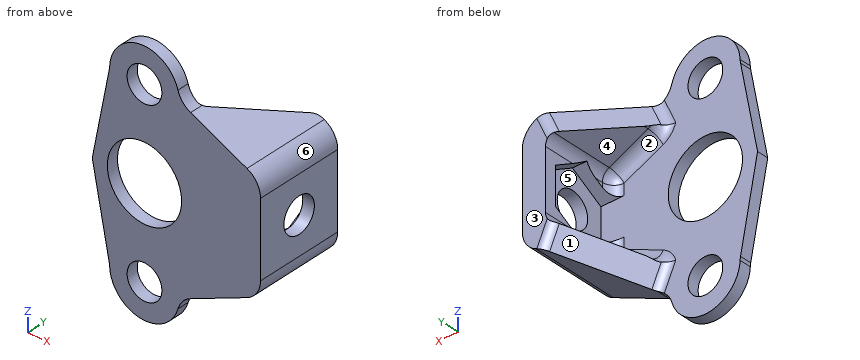
from build123d import *

# Parameters (mm, degrees)
ESQUISSE1_R                  = 3.2
ESQUISSE1_R_2                = 1.5
BOSS_EXTRU_1_DEPTH           = 1
BOSS_EXTRU_2_START           = 6.6
BOSS_EXTRU_2_DEPTH           = 6.6
CHANFREIN1_SIZE              = 6.6
CHANFREIN1_SIZE_2            = 4.73
CONG_1_R                     = 1
ENL_V_MAT_EXTRU_1_DEPTH      = 18.728508153
ENL_V_MAT_EXTRU_1_DEPTH_BACK = 1
ENL_V_MAT_EXTRU_2_DEPTH      = 18.728508153
ENL_V_MAT_EXTRU_2_DEPTH_BACK = 18.728508153
ESQUISSE2_3_R                = 1.5


with BuildPart() as part:
    # Esquisse1 → Boss.-Extru.1 (new body)
    # profile 1 of 2: a face of its own
    with BuildSketch(Plane(origin=(0, 0, 0), x_dir=(1, 0, 0), z_dir=(0, 1, 0))):
        with BuildLine():
            Line((7.41575976, 3.482294806), (4.054342249, 5.018942811))
            ThreePointArc((4.054342249, 5.018942811), (3.533019895, 5.579308264), (3.560627534, 6.344177047))
            Line((3.560627534, 6.344177047), (3.976387294, 7.253651523))
            ThreePointArc((3.976387294, 7.253651523), (3.291254041, 7.768850358), (2.884744089, 8.523560284))
            ThreePointArc((2.884744089, 8.523560284), (-0.351141019, 10.679379127), (-2.997167453, 7.830335178))
            ThreePointArc((-2.997167453, 7.830335178), (-3.009169797, 7.681917242), (-3.032181114, 7.534803614))
            Line((-3.032181114, 7.534803614), (-4.5, 0))
            Line((-4.5, 0), (-3.032181114, -7.534803614))
            ThreePointArc((-3.032181114, -7.534803614), (-3.009169797, -7.681917242), (-2.997167453, -7.830335178))
            ThreePointArc((-2.997167453, -7.830335178), (-0.351141019, -10.679379127), (2.884744089, -8.523560284))
            ThreePointArc((2.884744089, -8.523560284), (3.291254041, -7.768850358), (3.976387294, -7.253651523))
            Line((3.976387294, -7.253651523), (3.560627534, -6.344177047))
            ThreePointArc((3.560627534, -6.344177047), (3.533019895, -5.579308264), (4.054342249, -5.018942811))
            Line((4.054342249, -5.018942811), (7.41575976, -3.482294806))
            ThreePointArc((7.41575976, -3.482294806), (7.841355977, -3.113301708), (8, -2.572820331))
            Line((8, -2.572820331), (8, 2.572820331))
            ThreePointArc((8, 2.572820331), (7.841355977, 3.113301708), (7.41575976, 3.482294806))
        make_face()
        with Locations(Location((0, 0, 0), (0, 0, 270))):
            Circle(ESQUISSE1_R, mode=Mode.SUBTRACT)
        with Locations(Location((0, 7.7, 0), (0, 0, 270))):
            Circle(ESQUISSE1_R_2, mode=Mode.SUBTRACT)
        with Locations(Location((0, -7.7, 0), (0, 0, 270))):
            Circle(ESQUISSE1_R_2, mode=Mode.SUBTRACT)
    # profile 2 of 2: a face of its own
    with BuildSketch(Plane(origin=(0, 0, 0), x_dir=(1, 0, 0), z_dir=(0, 1, 0))):
        with BuildLine():
            ThreePointArc((4.054342249, 5.018942811), (3.533019895, 5.579308264), (3.560627534, 6.344177047))
            Line((3.560627534, 6.344177047), (3.976387294, 7.253651523))
            Line((3.976387294, 7.253651523), (8.831519521, 5.034162505))
            ThreePointArc((8.831519521, 5.034162505), (9.682711954, 4.29617631), (10, 3.215213554))
            Line((10, 3.215213554), (10, -3.215213554))
            ThreePointArc((10, -3.215213554), (9.682711954, -4.29617631), (8.831519521, -5.034162505))
            Line((8.831519521, -5.034162505), (3.976387294, -7.253651523))
            Line((3.976387294, -7.253651523), (3.560627534, -6.344177047))
            ThreePointArc((3.560627534, -6.344177047), (3.533019895, -5.579308264), (4.054342249, -5.018942811))
            Line((4.054342249, -5.018942811), (7.41575976, -3.482294806))
            ThreePointArc((7.41575976, -3.482294806), (7.841355977, -3.113301708), (8, -2.572820331))
            Line((8, -2.572820331), (8, 2.572820331))
            ThreePointArc((8, 2.572820331), (7.841355977, 3.113301708), (7.41575976, 3.482294806))
            Line((7.41575976, 3.482294806), (4.054342249, 5.018942811))
        make_face()
    extrude(amount=-BOSS_EXTRU_1_DEPTH)

    # Esquisse1<3> → Boss.-Extru.2 (add)
    with BuildSketch(Plane(origin=(0, 0, 0), x_dir=(1, 0, 0), z_dir=(0, 1, 0)).offset(BOSS_EXTRU_2_START)):
        with BuildLine():
            ThreePointArc((4.054342249, 5.018942811), (3.533019895, 5.579308264), (3.560627534, 6.344177047))
            Line((3.560627534, 6.344177047), (3.976387294, 7.253651523))
            Line((3.976387294, 7.253651523), (8.831519521, 5.034162505))
            ThreePointArc((8.831519521, 5.034162505), (9.682711954, 4.29617631), (10, 3.215213554))
            Line((10, 3.215213554), (10, -3.215213554))
            ThreePointArc((10, -3.215213554), (9.682711954, -4.29617631), (8.831519521, -5.034162505))
            Line((8.831519521, -5.034162505), (3.976387294, -7.253651523))
            Line((3.976387294, -7.253651523), (3.560627534, -6.344177047))
            ThreePointArc((3.560627534, -6.344177047), (3.533019895, -5.579308264), (4.054342249, -5.018942811))
            Line((4.054342249, -5.018942811), (7.41575976, -3.482294806))
            ThreePointArc((7.41575976, -3.482294806), (7.841355977, -3.113301708), (8, -2.572820331))
            Line((8, -2.572820331), (8, 2.572820331))
            ThreePointArc((8, 2.572820331), (7.841355977, 3.113301708), (7.41575976, 3.482294806))
            Line((7.41575976, 3.482294806), (4.054342249, 5.018942811))
        make_face()
    extrude(amount=-BOSS_EXTRU_2_DEPTH)

    # Chanfrein1
    # the kernel refuses this chamfer: 6.6, 4.73 mm, written as the material it takes off along each edge
    with BuildSketch(Plane(origin=(11.061264904, 6.6, 22.751821295), x_dir=(-0.020518924966706303, -0.9997454615139245, 0.009380079984775464), z_dir=(-0.4157597602676271, 0, -0.9094744755858766))) as chanfrein1_piece_1_section:
        Polygon((CHANFREIN1_SIZE * 0.999745461514, -CHANFREIN1_SIZE * 0.0225612983294), (-CHANFREIN1_SIZE_2 * 0.0225612983294, -CHANFREIN1_SIZE_2 * 0.999745461514), (0, 0), align=None)
    chanfrein1_piece_1 = extrude(amount=35.081593686, mode=Mode.PRIVATE)
    chanfrein1_piece_1 = split(chanfrein1_piece_1, bisect_by=Plane(origin=(5.170241743, 0, 6.158121449), z_dir=(0, 1, 0)), keep=Keep.TOP, mode=Mode.PRIVATE)
    add(chanfrein1_piece_1, mode=Mode.SUBTRACT)
    with BuildSketch(Plane(origin=(-3.524250076, 6.6, 9.153992725), x_dir=(-0.0205189249667065, -0.9997454615139245, -0.009380079984775552), z_dir=(0.4157597602676271, 0, -0.9094744755858766))) as chanfrein1_piece_2_section:
        Polygon((CHANFREIN1_SIZE * 0.999745461514, -CHANFREIN1_SIZE * 0.0225612983294), (-CHANFREIN1_SIZE_2 * 0.0225612983294, -CHANFREIN1_SIZE_2 * 0.999745461514), (0, 0), align=None)
    chanfrein1_piece_2 = extrude(amount=35.081593686, mode=Mode.PRIVATE)
    chanfrein1_piece_2 = split(chanfrein1_piece_2, bisect_by=Plane(origin=(5.170241743, 0, -6.158121449), z_dir=(0, 1, 0)), keep=Keep.TOP, mode=Mode.PRIVATE)
    add(chanfrein1_piece_2, mode=Mode.SUBTRACT)

    # Congé1
    cong_1_edges = [part.edges().sort_by_distance(p)[0] for p in [
        (7.862321613, 6.6, 4.377370464),
        (7.862321613, 6.6, -4.377370464),
        (3.768507414, 0, 6.798914285),
        (5.735051005, 0, 4.250618809),
        (7.841355977, 0, 3.113301708),
        (8, 0, 0),
        (7.841355977, 0, -3.113301708),
        (5.735051005, 0, -4.250618809),
        (3.768507414, 0, -6.798914285),
    ]]
    fillet(cong_1_edges, radius=CONG_1_R)

    # Esquisse2 → Enlèv. mat.-Extru.1 (cut, two sides: drawn at the far end of the back side and taken through both)
    with BuildSketch(Plane.ZY.offset(-8).offset(-ENL_V_MAT_EXTRU_1_DEPTH_BACK)):
        Polygon((3.233161507, 2.8), (1.616580754, 5.6), (-1.616580754, 5.6), (-3.233161507, 2.8), (-1.616580754, 0), (1.616580754, 0), align=None)
    extrude(amount=ENL_V_MAT_EXTRU_1_DEPTH + ENL_V_MAT_EXTRU_1_DEPTH_BACK, mode=Mode.SUBTRACT)

    # Esquisse2<3> → Enlèv. mat.-Extru.2 (cut, two sides: drawn at the far end of the back side and taken through both)
    with BuildSketch(Plane.ZY.offset(-8).offset(-ENL_V_MAT_EXTRU_2_DEPTH_BACK)):
        with Locations((0, 2.8)):
            Circle(ESQUISSE2_3_R)
    extrude(amount=ENL_V_MAT_EXTRU_2_DEPTH + ENL_V_MAT_EXTRU_2_DEPTH_BACK, mode=Mode.SUBTRACT)


solid = part.part
Source: CAD feature listing. Evaluate the final solid. Frame: model axes, mm. Face numbers are marked on the shaded views. A direction names the side the tool comes from. Give positions to 0.01 mm unless a question says otherwise; leave off trailing zeros. Write each loop counter-clockwise with the first axis right and the second up, starting at its lowest first coordinate (ties: lowest second). Pieces come first, ordered by that corner, then holes. Notation, with made-up numbers: M 33,-38.5 L 38,-38.5 A17 cw 38,-16.5 Z; hole C 85,34 d5. An arc over 180 degrees is marked long. Return JSON: item names as keys, results as strings. Group by question number.
1) Cut plane A-A, the plane x = 0. Output: boundary loops of the cut face in (y, z), then the cut area to 3 significant figures.
2) Cut plane C-C, the plane y = 5.25. Output: boundary loops of the cut face in (x, z).
3) Ray query, L1, parallel to X at y = 1.5, z = 1; L2, parallel to X at y = 5.75, z = 1.5; L3, parallel to Y at x = 5.25, z = -1.75. Return the intervals inside material, ascending.
4) First-contact query: pin 1 Ø2 at (x, y) = (7, 3) entering from -Z; pin 2 Ø4 at (x, z) = (1, 6) entering from +Y; pin 3 Ø2 at (y, z) = (5.5, 0.5) entering from -X. Flat tips, straight axial feed; report the tip coordinate or a pass-through.
5) Cut plane B-B, the plane y = 3.5. Output: boundary loops of the cut face in (x, z).
6) Set-up query: the marked faces 4, 5 and 6. Return all of +Z, -Z, +X, -X, +Y, -Y with unobstructed straight access to the full face (end or side cutting, diameter ignored); none if empty.
7) Draft query along Z for the marked faces 1, 2 and 3. Return one class per face: released by +Z, released by -Z, zero draft, split by the parting line, or undercut.
Data:
{
 "1": {"outline": "M -1,-10.7 L 0,-10.7 L 0,-9.2 L -1,-9.2 Z; M -1,-6.2 L 0,-6.2 L 0,-3.2 L -1,-3.2 Z; M -1,3.2 L 0,3.2 L 0,6.2 L -1,6.2 Z; M -1,9.2 L 0,9.2 L 0,10.7 L -1,10.7 Z", "area": "9.00 mm²"},
 "2": {"outline": "M 6.57,-3.87 L 7.4,-5.69 L 8.83,-5.03 A2 ccw 10,-3.22 L 10,3.22 A2 ccw 8.83,5.03 L 7.4,5.69 L 6.57,3.87 L 7.42,3.48 A1 cw 8,2.57 L 8,1.82 L 9,1.82 L 9,-1.82 L 8,-1.82 L 8,-2.57 A1 cw 7.42,-3.48 Z"},
 "3": {"L1": "x = 9 to 10", "L2": "x = 8 to 10", "L3": "y = -1 to 0"},
 "4": {"pin 1": "stops at z = -6.33", "pin 2": "stops at y = 0.05", "pin 3": "stops at x = 8"},
 "5": {"outline": "M 5.43,-4.39 L 6.26,-6.21 L 8.83,-5.03 A2 ccw 10,-3.22 L 10,-1.33 L 9,-1.33 L 9,-2.83 L 7.97,-2.83 A1 cw 7.42,-3.48 Z; M 5.43,4.39 L 7.42,3.48 A1 cw 7.97,2.83 L 9,2.83 L 9,1.33 L 10,1.33 L 10,3.22 A2 ccw 8.83,5.03 L 6.26,6.21 Z"},
 "6": {"face 4": "-X, +Y", "face 5": "-X", "face 6": "+Z, +X, +Y, -Y"},
 "7": {"face 1": "released by -Z", "face 2": "undercut", "face 3": "zero draft"}
}
